```python
from build123d import *

# Parameters (mm, degrees)
SKETCH1_W           = 22.225
SKETCH1_H           = 47.625
BOSS_EXTRUDE1_DEPTH = 30.1625
SKETCH2_R           = 14.2875
SKETCH2_R_2         = 2.5527
CUT_EXTRUDE1_DEPTH  = 45.393267367
CHAMFER1_SIZE       = 1.524


with BuildPart() as part:
    # Sketch1 → Boss-Extrude1 (new, symmetric)
    with BuildSketch(Plane(origin=(0, 0, 0), x_dir=(1, 0, 0), z_dir=(0, 1, 0))):
        Rectangle(SKETCH1_W, SKETCH1_H)
    extrude(amount=BOSS_EXTRUDE1_DEPTH, both=True)

    # Sketch2 → Cut-Extrude1 (cut, through all)
    with BuildSketch(Plane.ZY.offset(11.1125)):
        Circle(SKETCH2_R)
        with Locations((0, 25.4)):
            Circle(SKETCH2_R_2)
        with Locations((0, -25.4)):
            Circle(SKETCH2_R_2)
    extrude(amount=-CUT_EXTRUDE1_DEPTH, mode=Mode.SUBTRACT)

    # Chamfer1
    chamfer1_edges = [part.edges().sort_by_distance(p)[0] for p in [
        (11.1125, 30.1625, 0),
        (0, 30.1625, -23.8125),
        (-11.1125, 30.1625, 0),
        (0, -30.1625, -23.8125),
        (11.1125, -30.1625, 0),
        (0, -30.1625, 23.8125),
        (-11.1125, -30.1625, 0),
        (-11.1125, 0, -23.8125),
        (11.1125, 0, -23.8125),
        (11.1125, 0, 23.8125),
        (-11.1125, 0, 23.8125),
        (0, 30.1625, 23.8125),
    ]]
    chamfer(chamfer1_edges, length=CHAMFER1_SIZE)


solid = part.part
```
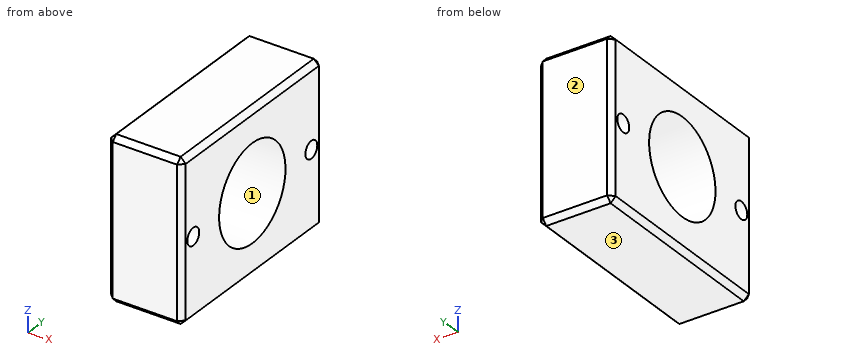
Can you work these out from the model? Positions are in its coordinate system, mm. Face numbers are marked on the shaded views. Give positions to 0.01 mm unless a question says otherwise; leave off trailing zeros. Write each loop counter-clockwise with the first axis right and the second up, starting at its lowest first coordinate (ties: lowest second). Pieces come first, ordered by that corner, then holes. Notation, with made-up numbers: (-39.5, 4.25) - (-12.5, 4.25) arc R24 cw to (-12.5, 31.25) - close; hole circle Ø8 at (18.5, 4.5). An arc over 180 degrees is marked (long way). Write item = value, one per line. Start each with the question number.
1. Imagine slicing it at C-C (x = 1). Please give me the cut outline in (y, z) (1 decimal).
2. Please list where these lines run through material, in increasing order: line 1 (Y direction, x = -3.5, z = 0); line 2 (Z direction, x = -1, y = -0.5); line 3 (Z direction, x = 10, y = 11.5).
3. Imagine slicing it at B-B (y = 0). Please give me the cut outline in (x, z), and give its area (3 significant figures).
4. Imagine slicing it at A-A (z = 0). Please give me the cut outline in (x, y).
5. Thinking about a two-plate mould opening in Z: for the marked faces 1, 2 and 3, which applies, released by +Z, released by -Z, zero draft, split by the parting line, or undercut?
6. Imagine slicing it at D-D (z = 6.5). Please give me the cut outline in (x, y).
Worked answers:
q1.outline = (-30.2, -22.3) - (-28.6, -23.8) - (28.6, -23.8) - (30.2, -22.3) - (30.2, 22.3) - (28.6, 23.8) - (-28.6, 23.8) - (-30.2, 22.3) - close; hole circle Ø5.1 at (-25.4, 0); hole circle Ø28.6 at (0, 0); hole circle Ø5.1 at (25.4, 0)
q2.line_1 = -30.16 to -27.95, -22.85 to -14.29, 14.29 to 22.85, 27.95 to 30.16
q2.line_2 = -23.81 to -14.28, 14.28 to 23.81
q2.line_3 = -23.4 to -8.48, 8.48 to 23.4
q3.outline = (-11.11, -22.29) - (-9.59, -23.81) - (9.59, -23.81) - (11.11, -22.29) - (11.11, -14.29) - (-11.11, -14.29) - close; (-11.11, 14.29) - (11.11, 14.29) - (11.11, 22.29) - (9.59, 23.81) - (-9.59, 23.81) - (-11.11, 22.29) - close
q3.area = 419 mm2
q4.outline = (-11.11, -28.64) - (-9.59, -30.16) - (9.59, -30.16) - (11.11, -28.64) - (11.11, -27.95) - (-11.11, -27.95) - close; (-11.11, -22.85) - (11.11, -22.85) - (11.11, -14.29) - (-11.11, -14.29) - close; (-11.11, 14.29) - (11.11, 14.29) - (11.11, 22.85) - (-11.11, 22.85) - close; (-11.11, 27.95) - (11.11, 27.95) - (11.11, 28.64) - (9.59, 30.16) - (-9.59, 30.16) - (-11.11, 28.64) - close
q5.face_1 = undercut
q5.face_2 = zero draft
q5.face_3 = released by -Z
q6.outline = (-11.11, -28.64) - (-9.59, -30.16) - (9.59, -30.16) - (11.11, -28.64) - (11.11, -12.72) - (-11.11, -12.72) - close; (-11.11, 12.72) - (11.11, 12.72) - (11.11, 28.64) - (9.59, 30.16) - (-9.59, 30.16) - (-11.11, 28.64) - close
